```python
from build123d import *

# Parameters (mm, degrees)
ESQUISSE1_W              = 80
ESQUISSE1_H              = 40
BOSS_EXTRU_1_DEPTH       = 6
ESQUISSE9_R              = 2.5
ESQUISSE9_R_2            = 2.3
ENL_V_MAT_EXTRU_12_DEPTH = 35


with BuildPart() as part:
    # Esquisse1 → Boss.-Extru.1 (new body)
    with BuildSketch(Plane(origin=(0, 0, 0), x_dir=(1, 0, 0), z_dir=(0, 1, 0))):
        Polygon((-150, 0), (-150, 260), (-110, 300), (110, 300), (150, 260), (150, 0), align=None)
        with Locations((0, 75)):
            Rectangle(ESQUISSE1_W, ESQUISSE1_H, mode=Mode.SUBTRACT)
        with Locations((0, 225)):
            Rectangle(ESQUISSE1_W, ESQUISSE1_H, mode=Mode.SUBTRACT)
    extrude(amount=BOSS_EXTRU_1_DEPTH)

    # Esquisse9 → Enlèv. mat.-Extru.12 (cut)
    with BuildSketch(Plane(origin=(0, 6, 0), x_dir=(1, 0, 0), z_dir=(0, 1, 0))):
        with Locations(Location((-100, 249.602322281, 0), (0, 0, 270))):
            Circle(ESQUISSE9_R)
        with Locations(Location((-75.031111773, 223.085817986, 0), (0, 0, 270))):
            Circle(ESQUISSE9_R)
        with Locations(Location((73.483495706, 223.085817986, 0), (0, 0, 270))):
            Circle(ESQUISSE9_R)
        with Locations(Location((100, 249.602322281, 0), (0, 0, 270))):
            Circle(ESQUISSE9_R)
        with Locations(Location((73.483495706, 72.865212221, 0), (0, 0, 270))):
            Circle(ESQUISSE9_R)
        with Locations(Location((100, 49.602322281, 0), (0, 0, 270))):
            Circle(ESQUISSE9_R)
        with Locations(Location((-73.489446443, 74.470995042, 0), (0, 0, 270))):
            Circle(ESQUISSE9_R_2)
        with Locations(Location((-100, 49.602322281, 0), (0, 0, 270))):
            Circle(ESQUISSE9_R)
    extrude(amount=-ENL_V_MAT_EXTRU_12_DEPTH, mode=Mode.SUBTRACT)


solid = part.part
```
The listing builds one solid part. Answer for the finished solid, in the listing's coordinates (mm). Give positions to 0.01 mm unless a question says otherwise; leave off trailing zeros. Loops run counter-clockwise (first coordinate to the right, second up) from the corner with the lowest first, then second, coordinate; pieces in that order, holes last. Notation, with made-up numbers: (72.5, 36) - (129.5, 36) arc R12 ccw to (129.5, 54) - close; hole circle Ø6 at (40.5, 32.25). An arc over 180 degrees is marked (long way). Return JSON: item names as keys, results as strings. Group by question number.
1. Find section A-A (y = 2.45). State how many separate pieces and enclosed holes the cut face has, then the cut area to 3 significant figures.
2. Determine the mould class of faces 1 (the flat face through (2, 0, -152)), 2 (the flat face through (130, 3, -280)) for opening direction Z: pulls with the +Z half, pulls with the -Z half, needs draft (parallel to the pull), parting line crosses it, or undercut.
3. Given pin 1 Ø4.5 at (x, z) = (73.48, -72.87) entering from -Y, flat-ended and moving along its own axis, determine where the tip first touches the part or whether it passes through.
4. Find section B-B (z = -280). Write down the section's boundary in (x, y), then the cut area to 3 significant figures.
5. Straight lines are drawn through the part: line 1 (Z direction, x = -13, y = 1.3); line 2 (X direction, y = 5, z = -238); line 3 (Z direction, x = -74.5, y = 5.3). For each, find the intervals that lie inside material, in ascending order. Write a range as [from, to].
Verdict:
{
 "1": {"separate pieces": "1", "enclosed holes": "10", "area": "81,800 mm^2"},
 "2": {"face 1": "needs draft", "face 2": "pulls with the -Z half"},
 "3": {"pin 1": "passes through"},
 "4": {"outline": "(-130, 0) - (130, 0) - (130, 6) - (-130, 6) - close", "area": "1,560 mm^2"},
 "5": {"line 1": "z = [-300, -245], [-205, -95], [-55, 0]", "line 2": "x = [-150, -40], [40, 150]", "line 3": "z = [-300, -225.53], [-220.64, -76.54], [-72.4, 0]"}
}
